Check sheet for the modelled part. Datum: model origin and axes. Units: mm. A direction names the side the tool comes from. Give positions to 0.01 mm unless a question says otherwise; leave off trailing zeros. Loops run counter-clockwise (first coordinate to the right, second up) from the corner with the lowest first, then second, coordinate; pieces in that order, holes last. Notation, with made-up numbers: M -3,32 L 48,32 A19 cw 48,69 Z; hole C 80.5,76.25 d9. An arc over 180 degrees is marked long. Use one line per item in the form item = value.
from build123d import *

# Parameters (mm, degrees)
PAD_DEPTH                = 1.2
SKETCH001_R              = 3.15
PAD001_DEPTH             = 3
SKETCH002_R              = 0.8
POCKET_DEPTH             = 4.201
SKETCH003_R              = 1.5
POCKET001_DEPTH          = 5
CLONE002_PLACEMENT_ANGLE = -90


with BuildPart() as part:
    # Sketch → Pad (new body)
    with BuildSketch(Plane.XY):
        with BuildLine():
            ThreePointArc((-19.975767, 27.046834), (-27.046834, 27.046834), (-27.046834, 19.975767))
            Line((-23.375519, 16.304451), (-27.046834, 19.975767))
            ThreePointArc((-16.304451, 23.375519), (-20.152543, 20.152543), (-23.375519, 16.304451))
            Line((-19.975767, 27.046834), (-16.304451, 23.375519))
        make_face()
    extrude(amount=PAD_DEPTH)

    # Sketch001 → Pad001 (new body)
    with BuildSketch(Plane.XY.offset(1.2)):
        with Locations((-23.5113, 23.5113)):
            Circle(SKETCH001_R)
    extrude(amount=PAD001_DEPTH)

    # Sketch002 → Pocket (cut, through all)
    with BuildSketch(Plane.XY.offset(4.2)):
        with Locations((-23.5113, 23.5113)):
            Circle(SKETCH002_R)
    extrude(amount=-POCKET_DEPTH, mode=Mode.SUBTRACT)

    # Sketch003 → Pocket001 (cut)
    with BuildSketch(Plane.XY.offset(4.2)):
        with Locations((-23.5113, 23.5113)):
            Circle(SKETCH003_R)
    extrude(amount=-POCKET001_DEPTH, mode=Mode.SUBTRACT)


with BuildPart() as part_1:
    # Clone002 placement: moved
    add(part.part.rotate(Axis((0, 0, 0), (0, 0, 1)), CLONE002_PLACEMENT_ANGLE))


solid = part_1.part
1) Section check C-C (x = 25.5). Record the cut outline in (y, z), then the cut area to 3 significant figures.
Evaluation:
outline = M 18.43,0 L 28.1,0 L 28.1,1.2 L 25.95,1.2 L 25.95,4.2 L 21.07,4.2 L 21.07,1.2 L 18.43,1.2 Z
area = 26.3 mm^2
2) Release check for a two-part mould opening along X. For faces 1 (the face through (20.436, 24.194, 2.679)), 2 (the face through (20.202, 20.103, 0.592)), 3 (the face through (22.937, 22.126, 2.129)) record: pulls with the +X half, pulls with the -X half, needs draft (parallel to the pull), parting line crosses it, or undercut.
Evaluation:
face_1 = parting line crosses it
face_2 = pulls with the -X half
face_3 = undercut
3) Depth check by flat-ended pin: pin 1 Ø2 at (x, y) = (26.5, 20.5) entering from +Z; pin 2 Ø2 at (y, z) = (21.5, 1.5) entering from +X. Enter the tip coordinate at first touch or a pass-through.
Evaluation:
pin_1 = 1.2
pin_2 = 28.4
4) Section check A-A (y = 22.5). Record the cut outline in (x, z).
Evaluation:
outline = M 17.49,0 L 22.4,0 L 22.4,4.2 L 20.53,4.2 L 20.53,1.2 L 17.49,1.2 Z; M 24.62,0 L 28.41,0 L 28.41,1.2 L 26.49,1.2 L 26.49,4.2 L 24.62,4.2 Z
5) Section check D-D (z = 3.3). Record the cut outline in (x, y).
Evaluation:
outline = C 23.51,23.51 d6.3; hole C 23.51,23.51 d3
6) Section check B-B (x = 24.25). Record the cut outline in (y, z), then the cut area to 3 significant figures.
Evaluation:
outline = M 17.18,0 L 22.21,0 L 22.21,4.2 L 20.45,4.2 L 20.45,1.2 L 17.18,1.2 Z; M 24.82,0 L 28.46,0 L 28.46,1.2 L 26.57,1.2 L 26.57,4.2 L 24.82,4.2 Z
area = 20.9 mm^2
7) Scan lines: line 1 (Y direction, x = 23.5, z = 2.25); line 2 (X direction, y = 22.5, z = 2.05). Record each from-to range of solid material in increasing order.
Evaluation:
line_1 = 20.36 to 22.01, 25.01 to 26.66
line_2 = 20.53 to 22.4, 24.62 to 26.49
8) Set-up check for faces 4 (the face through (21, 21, 1.2)), 5 (the face through (27.12, 26.97, 0.59)): record each of +Z, -Z, +X, -X, +Y, -Y from which the full face is reachable in a straight line by a thin tool's end or side.
Evaluation:
face_4 = +Z
face_5 = +Z, -Z
